from build123d import *

# Parameters (mm, degrees)
CROQUIS1_R              = 35
CROQUIS1_R_2            = 31
SALIENTE_EXTRUIR1_DEPTH = 70
CROQUIS2_R              = 31
SALIENTE_EXTRUIR2_DEPTH = 55


with BuildPart() as part:
    # Croquis1 → Saliente-Extruir1 (new body)
    with BuildSketch(Plane.XY):
        Circle(CROQUIS1_R)
        Circle(CROQUIS1_R_2, mode=Mode.SUBTRACT)
    extrude(amount=SALIENTE_EXTRUIR1_DEPTH)

    # Croquis2 → Saliente-Extruir2 (add)
    with BuildSketch(Plane(origin=(0, 0, 0), x_dir=(-1, 0, 0), z_dir=(0, 0, -1))):
        Circle(CROQUIS2_R)
    extrude(amount=-SALIENTE_EXTRUIR2_DEPTH)

    # Cortar-Recubrir2: read off the stored shape, not the designer's step
    # Cortar-Recubrir2: loft between two sections, ruled curve by curve
    cortar_recubrir2_from = [
        Edge.make_bspline([(24.505743897, 4.946566089, 55), (34.398876075, -44.064921704, 55), (-14.612611719, -53.958053882, 55), (-24.505743897, -4.946566089, 55), (-34.398876075, 44.064921704, 55), (14.612611719, 53.958053882, 55), (24.505743897, 4.946566089, 55)], [0, 0, 0, 0, 0.5, 0.5, 0.5, 1, 1, 1, 1], 3, [1, 0.333333333, 0.333333333, 1, 0.333333333, 0.333333333, 1]),
    ]
    cortar_recubrir2_to = [
        Edge.make_bspline([(10.528812483, 15.875975803, 0), (42.280764089, -5.181649163, 0), (21.223139123, -36.933600769, 0), (-10.528812483, -15.875975803, 0), (-42.280764089, 5.181649163, 0), (-21.223139123, 36.933600769, 0), (10.528812483, 15.875975803, 0)], [0, 0, 0, 0, 0.5, 0.5, 0.5, 1, 1, 1, 1], 3, [1, 0.333333333, 0.333333333, 1, 0.333333333, 0.333333333, 1]),
    ]
    cortar_recubrir2 = Solid(Shell([*[Face.make_surface_from_curves(cortar_recubrir2_from[k], cortar_recubrir2_to[k]) for k in range(1)], Face(Wire(cortar_recubrir2_from)), Face(Wire(cortar_recubrir2_to))]))
    add(cortar_recubrir2, mode=Mode.SUBTRACT)


solid = part.part
Input: part model. Units: mm. Frame: model coordinates. A direction names the side the tool comes from. Round coordinates to 2 decimals unless told otherwise and drop trailing zeros. Order: outer loops, then holes, each group sorted by start corner. A loop starts at its lowest first (then second) coordinate and runs counter-clockwise, first axis right, second up. Notation, with made-up numbers: (-20, 0.5) - (23, 0.5) arc R30 ccw to (23, 31.5) - close; hole circle Ø8 at (78, 15.25). An arc over 180 degrees is marked (long way). Answer as a JSON object with one key per item and string values. Group by question number.
(1) Material intervals for probe 1 along Y at (x, z) = (0, 59.75); probe 2 along Y at (x, z) = (28.5, 64); probe 3 along Z at (x, y) = (-28, -8.5), sorted ascending. Write a range as from..to.
(2) Pin query (flat end, axial travel): P1, Ø10, axis at y = -25, z = 46.5, coming from the +X side; P2, Ø5, axis at y = 7, z = 34, coming from the -X side; P3, Ø12, axis at y = -19.5, z = 12.5, coming from the +X side. Return the tip coordinate at first contact, or that it passes through.
(3) Cut plane B-B (x = -29.5). Return loops of the section in (y, z), then the cut area to 3 significant figures.
(4) Cut plane A-A (z = 58.5). Return loops of the section in (x, y).
(5) Draft query along X for faces 1 (the face through (-28, -21, 35)), 2 (the face through (10, 17, 0)), 3 (the face through (8, 24, 55)). Return one class per face: released by +X, released by -X, zero draft, split by the parting line, or undercut.
(6) Reachability of faces 4 (the face through (-20.9, -23.2, 70)), 5 (the face through (-4.036, 30.736, 62.395)) from +Z, -Z, +X, -X, +Y, -Y: full face, straight path, thin tool, end or side. Return the list, or none.
Here are the results:
{
 "1": {"probe 1": "y = -35..-31, 31..35", "probe 2": "y = -20.32..-12.2, 12.2..20.32", "probe 3": "z = 0..55"},
 "2": {"P1": "stops at x = 28.72", "P2": "stops at x = -34.71", "P3": "stops at x = 32.29"},
 "3": {"outline": "(-18.83, 0) - (18.83, 0) - (18.83, 70) - (9.53, 70) - (9.53, 55) - (-9.53, 55) - (-9.53, 70) - (-18.83, 70) - close", "area": "2,350 mm^2"},
 "4": {"outline": "circle Ø70 at (0, 0); hole circle Ø62 at (0, 0)"},
 "5": {"face 1": "split by the parting line", "face 2": "zero draft", "face 3": "undercut"},
 "6": {"face 4": "+Z, +X, -X, +Y, -Y", "face 5": "+Z"}
}
